Work out the finished part from the listing and answer in its coordinate system (mm). Round coordinates to 2 decimals unless told otherwise and drop trailing zeros. Write each loop counter-clockwise with the first axis right and the second up, starting at its lowest first coordinate (ties: lowest second). Pieces come first, ordered by that corner, then holes.
from build123d import *

# Parameters (mm, degrees)
SKETCH_1_R          = 50
EXTRUDE_1_DEPTH     = 5
SKETCH_4_R          = 7.5
CUT_EXTRUDE_3_DEPTH = 10
SKETCH_5_R          = 2
CUT_EXTRUDE_4_DEPTH = 10
SKETCH_6_R          = 3.38
CUT_EXTRUDE_5_DEPTH = 71.887234394


with BuildPart() as part:
    # 스케치1 → 보스-돌출1 (new body)
    with BuildSketch(Plane.XY):
        Circle(SKETCH_1_R)
    extrude(amount=EXTRUDE_1_DEPTH)

    # 스케치4 → 컷-돌출3 (cut)
    with BuildSketch(Plane.XY.offset(5)):
        Circle(SKETCH_4_R)
    extrude(amount=-CUT_EXTRUDE_3_DEPTH, mode=Mode.SUBTRACT)

    # 스케치5 → 컷-돌출4 (cut)
    with BuildSketch(Plane.XY.offset(5)):
        with Locations((-23, 8)):
            Circle(SKETCH_5_R)
        with Locations((23, 8)):
            Circle(SKETCH_5_R)
        with Locations((23, -8)):
            Circle(SKETCH_5_R)
        with Locations((-23, -8)):
            Circle(SKETCH_5_R)
    extrude(amount=-CUT_EXTRUDE_4_DEPTH, mode=Mode.SUBTRACT)

    # 스케치6 → 컷-돌출5 (cut, through all)
    with BuildSketch(Plane.XY.offset(5)):
        with Locations((0, 50)):
            Circle(SKETCH_6_R)
        with Locations((8.682408883, 49.240387651)):
            Circle(SKETCH_6_R)
        with Locations((17.101007166, 46.984631039)):
            Circle(SKETCH_6_R)
        with Locations((25, 43.301270189)):
            Circle(SKETCH_6_R)
        with Locations((32.139380484, 38.302222156)):
            Circle(SKETCH_6_R)
        with Locations((38.302222156, 32.139380484)):
            Circle(SKETCH_6_R)
        with Locations((43.301270189, 25)):
            Circle(SKETCH_6_R)
        with Locations((46.984631039, 17.101007166)):
            Circle(SKETCH_6_R)
        with Locations((49.240387651, 8.682408883)):
            Circle(SKETCH_6_R)
        with Locations((50, 0)):
            Circle(SKETCH_6_R)
        with Locations((49.240387651, -8.682408883)):
            Circle(SKETCH_6_R)
        with Locations((46.984631039, -17.101007166)):
            Circle(SKETCH_6_R)
        with Locations((43.301270189, -25)):
            Circle(SKETCH_6_R)
        with Locations((38.302222156, -32.139380484)):
            Circle(SKETCH_6_R)
        with Locations((32.139380484, -38.302222156)):
            Circle(SKETCH_6_R)
        with Locations((25, -43.301270189)):
            Circle(SKETCH_6_R)
        with Locations((17.101007166, -46.984631039)):
            Circle(SKETCH_6_R)
        with Locations((8.682408883, -49.240387651)):
            Circle(SKETCH_6_R)
        with Locations((0, -50)):
            Circle(SKETCH_6_R)
        with Locations((-8.682408883, -49.240387651)):
            Circle(SKETCH_6_R)
        with Locations((-17.101007166, -46.984631039)):
            Circle(SKETCH_6_R)
        with Locations((-25, -43.301270189)):
            Circle(SKETCH_6_R)
        with Locations((-32.139380484, -38.302222156)):
            Circle(SKETCH_6_R)
        with Locations((-38.302222156, -32.139380484)):
            Circle(SKETCH_6_R)
        with Locations((-43.301270189, -25)):
            Circle(SKETCH_6_R)
        with Locations((-46.984631039, -17.101007166)):
            Circle(SKETCH_6_R)
        with Locations((-49.240387651, -8.682408883)):
            Circle(SKETCH_6_R)
        with Locations((-50, 0)):
            Circle(SKETCH_6_R)
        with Locations((-49.240387651, 8.682408883)):
            Circle(SKETCH_6_R)
        with Locations((-46.984631039, 17.101007166)):
            Circle(SKETCH_6_R)
        with Locations((-43.301270189, 25)):
            Circle(SKETCH_6_R)
        with Locations((-38.302222156, 32.139380484)):
            Circle(SKETCH_6_R)
        with Locations((-32.139380484, 38.302222156)):
            Circle(SKETCH_6_R)
        with Locations((-25, 43.301270189)):
            Circle(SKETCH_6_R)
        with Locations((-17.101007166, 46.984631039)):
            Circle(SKETCH_6_R)
        with Locations((-8.682408883, 49.240387651)):
            Circle(SKETCH_6_R)
    extrude(amount=-CUT_EXTRUDE_5_DEPTH, mode=Mode.SUBTRACT)


solid = part.part
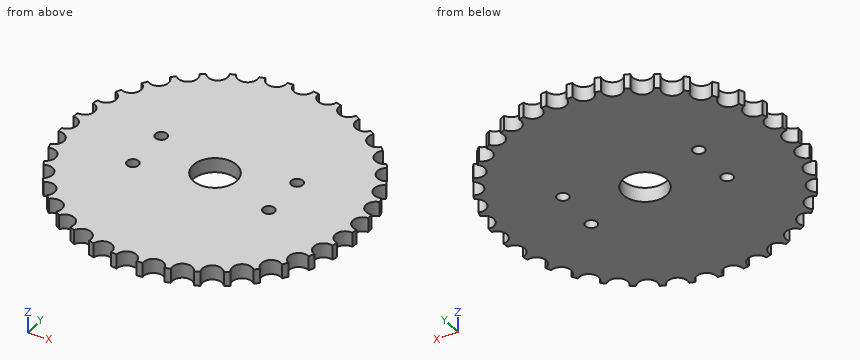
Q1. Find section A-A (x = 0). Determine the outline of the cut face in (y, z), plus the area to 3 significant figures.
Q2. Find section C-C (z = 2.15). Count the separate pieces of the cut face and the enclosed holes in it, plus the area to 3 significant figures.
Q3. Given pin 1 (3.5 mm diameter, centred on x = 23, y = -8, fed in from +Z); pin 2 (3 mm diameter, centred on x = -8.5, z = 4, fed in from -Y); pin 3 (2 mm diameter, centred on y = -7.5, z = 1, fed in from +X); pin 4 (3 mm diameter, centred on x = -28.5, z = 4, fed in from +Y), each flat-ended and moving along its own axis, determine where each tip first touches the part or whether it passes through.
Q4. Find the intervals of material crossed by L1, parallel to Y at x = -23, z = 1.9; L2, parallel to X at y = 9, z = 3.9; L3, parallel to Y at x = 41, z = 2.85, in increasing order.
Q5. Find section D-D (x = 19). Determine the outline of the cut face in (y, z), plus the area to 3 significant figures.
Report:
1. outline: (-46.62, 0) - (-7.5, 0) - (-7.5, 5) - (-46.62, 5) - close; (7.5, 0) - (46.62, 0) - (46.62, 5) - (7.5, 5) - close
1. area: 391 mm2
2. separate pieces: 1
2. enclosed holes: 5
2. area: 6,990 mm2
3. pin 1: passes through
3. pin 2: stops at y = -46.31
3. pin 3: stops at x = 46.66
3. pin 4: stops at y = 41.51
4. L1: y = -40.58 to -10, -6 to 6, 10 to 40.58
4. L2: x = -45.88 to -24.73, -21.27 to 21.27, 24.73 to 45.88
4. L3: y = -28.62 to -27.48, -22.52 to 22.52, 27.48 to 28.62
5. outline: (-44.19, 0) - (44.19, 0) - (44.19, 5) - (-44.19, 5) - close
5. area: 442 mm2
